For this review, take the finished solid that the model builds, in its own axes (mm). A direction names the side the tool comes from. Coordinates: 2 decimals unless noted, no trailing zeros. Write each loop counter-clockwise with the first axis right and the second up, starting at its lowest first coordinate (ties: lowest second). Pieces come first, ordered by that corner, then holes. Notation, with made-up numbers: M 3.5,69.5 L 60.5,69.5 A22 cw 60.5,96.5 Z; hole C 5.25,-3 d5. An arc over 180 degrees is marked long. One line per question, with ' | ' between items.
from build123d import *

# Parameters (mm, degrees)
SKETCH1_W                  = 50
SKETCH1_H                  = 38
MAIN_BODY_DEPTH            = 10
SIDE_MOUNTING_BODY_DEPTH   = 2
F_3_1_3_1_DIAMETER_HOLE1_D = 3.1
SKETCH5_W                  = 48
SKETCH5_H                  = 18
BOTTOM_CUT_DEPTH           = 2.6
SKETCH6_W                  = 50
SKETCH6_H                  = 1
BOTTOM_MOUNTING_TAB_DEPTH  = 15
SLOT_DEPTH                 = 2
FILLET1_R                  = 1.5
FILLET2_R                  = 3


with BuildPart() as part:
    # Sketch1 → MAIN BODY (new body, symmetric)
    with BuildSketch(Plane.XY):
        Rectangle(SKETCH1_W, SKETCH1_H)
    extrude(amount=MAIN_BODY_DEPTH, both=True)

    # Sketch2 → SIDE MOUNTING BODY (add)
    with BuildSketch(Plane(origin=(0, 0, -10), x_dir=(-1, 0, 0), z_dir=(0, 0, -1))):
        with BuildLine():
            Line((30.959543616, -2.332441235), (25, -9))
            Line((25, -9), (25, 9))
            Line((25, 9), (30.959543616, 2.332441235))
            ThreePointArc((30.959543616, 2.332441235), (31.85, 0), (30.959543616, -2.332441235))
        make_face()
    side_mounting_body = extrude(amount=-SIDE_MOUNTING_BODY_DEPTH)

    # Mirror1: SIDE MOUNTING BODY across plane
    add(side_mounting_body.mirror(Plane(origin=(0, 0, 0), x_dir=(0, 0, 1), z_dir=(1, 0, 0))))

    # Ø3.1 (3.1) Diameter Hole1 (through all)
    with Locations(Plane.XY.offset(-8)):
        with Locations((-28.35, 0), (28.35, 0)):
            Hole(F_3_1_3_1_DIAMETER_HOLE1_D / 2)

    # Sketch5 → BOTTOM CUT (cut)
    with BuildSketch(Plane(origin=(0, -19, 0), x_dir=(-1, 0, 0), z_dir=(0, -1, 0))):
        Rectangle(SKETCH5_W, SKETCH5_H)
    extrude(amount=-BOTTOM_CUT_DEPTH, mode=Mode.SUBTRACT)

    # Sketch6 → BOTTOM MOUNTING TAB (add)
    with BuildSketch(Plane(origin=(0, -19, 0), x_dir=(-1, 0, 0), z_dir=(0, -1, 0))):
        with Locations((0, 9.5)):
            Rectangle(SKETCH6_W, SKETCH6_H)
    extrude(amount=BOTTOM_MOUNTING_TAB_DEPTH)

    # Sketch7 → SLOT (cut, through all)
    with BuildSketch(Plane.XY.offset(-9)):
        with BuildLine():
            Line((-19.45, -24.85), (-19.45, -27.95))
            ThreePointArc((-19.45, -27.95), (-21, -29.5), (-22.55, -27.95))
            Line((-22.55, -27.95), (-22.55, -24.85))
            ThreePointArc((-22.55, -24.85), (-21, -23.3), (-19.45, -24.85))
        make_face()
    slot = extrude(amount=-SLOT_DEPTH, mode=Mode.SUBTRACT)

    # Mirror2: SLOT across plane
    add(slot.mirror(Plane(origin=(0, 0, 0), x_dir=(0, 0, 1), z_dir=(1, 0, 0))), mode=Mode.SUBTRACT)

    # Fillet1
    fillet1_edges = [part.edges().sort_by_distance(p)[0] for p in [
        (24, -16.4, 0),
        (24, -17.7, 9),
        (0, -16.4, -9),
        (24, -17.7, -9),
        (-24, -16.4, 0),
        (-24, -17.7, -9),
        (0, -16.4, 9),
        (-24, -17.7, 9),
    ]]
    fillet(fillet1_edges, radius=FILLET1_R)

    # Fillet2
    fillet2_edges = [part.edges().sort_by_distance(p)[0] for p in [
        (25, -34, -9.5),
        (-25, -34, -9.5),
    ]]
    fillet(fillet2_edges, radius=FILLET2_R)


solid = part.part
1. Draft analysis for pull direction Z (two halves, no side actions). For faces 1 (the flat face through (0, -16.4, 0)), 2 (the flat face through (-9.4, -19, 9.7)), state which applies: pulls with the +Z half, pulls with the -Z half, needs draft (parallel to the pull), parting line crosses it, or undercut.
Computed values:
face 1: undercut | face 2: needs draft
2. Machinability: for faces 3 (the cylindrical face through (-21, -23.3, -9.5)), 4 (the cylindrical face through (23.57, -16.85, -0.11)), 5 (the flat face through (0, 19, 0)), which of the approach directions +Z, -Z, +X, -X, +Y, -Y give a long, thin tool a straight path to every point of the face, cutting with its end or side? Answer none if there is none.
Computed values:
face 3: +Z, -Z | face 4: -Y | face 5: +Z, -Z, +X, -X, +Y
3. For line 1 along Y through (x, z) = (-22, 7.5); line 2 along X through (y, z) = (8.5, 8.25); line 3 along Y through (x, z) = (-28.35, -8.75), list the stretches that pass through material, from the lowest coordinate up.
Computed values:
line 1: y = -16.4 to 19 | line 2: x = -25 to 25 | line 3: y = -5.25 to -1.55, 1.55 to 5.25
4. Clearance check with flat-ended pins moving along their axes: P1, Ø1.1, axis at y = -27, z = -9.5, coming from the -X side; P2, Ø17.5, axis at x = -5.5, y = -30, coming from the +Z side; P3, Ø2, axis at x = -28.5, y = -2.5, coming from the +Z side. State where each tip first meets the part, or that it passes through.
Computed values:
P1: stops at x = -25 | P2: stops at z = -9 | P3: stops at z = -8
5. Take a section at C-C on x = 11.5. State the section outline as (y, z) points, plus the area to 3 significant figures.
Computed values:
outline: M -34,-10 L 19,-10 L 19,10 L -19,10 L -19,9 L -17.9,9 A1.5 cw -16.4,7.5 L -16.4,-7.5 A1.5 cw -17.9,-9 L -34,-9 Z | area: 729 mm2
6. Take a section at A-A on x = 21. State the section outline as (y, z) points, plus the area to 3 significant figures.
Computed values:
outline: M -34,-10 L -29.5,-10 L -29.5,-9 L -34,-9 Z; M -23.3,-10 L 19,-10 L 19,10 L -19,10 L -19,9 L -17.9,9 A1.5 cw -16.4,7.5 L -16.4,-7.5 A1.5 cw -17.9,-9 L -23.3,-9 Z | area: 723 mm2
7. Take a section at B-B on y = -26. State the section outline as (x, z) points.
Computed values:
outline: M -25,-10 L -22.55,-10 L -22.55,-9 L -25,-9 Z; M -19.45,-10 L 19.45,-10 L 19.45,-9 L -19.45,-9 Z; M 22.55,-10 L 25,-10 L 25,-9 L 22.55,-9 Z
8. Take a section at D-D on z = 1.5. State the section outline as (x, y) points.
Computed values:
outline: M -25,-19 L -24,-19 L -24,-17.9 A1.5 cw -22.5,-16.4 L 22.5,-16.4 A1.5 cw 24,-17.9 L 24,-19 L 25,-19 L 25,19 L -25,19 Z
